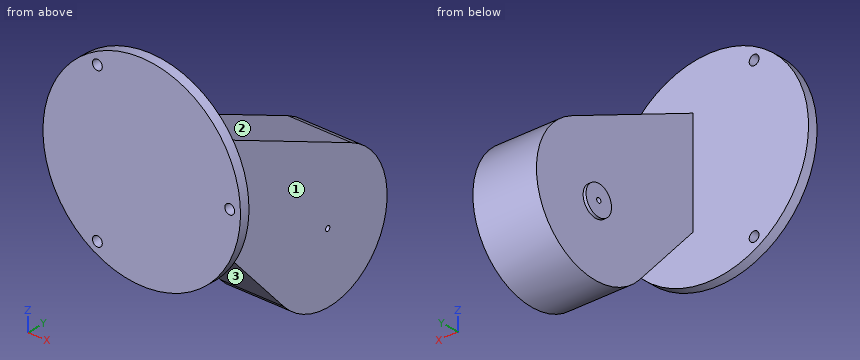
```python
from build123d import *

# Parameters (mm, degrees)
SKETCH_1_R               = 101
EXTRUDE_1_DEPTH          = 10
SKETCH_2_R               = 5
CUT_EXTRUDE_1_DEPTH      = 144.185194765
PATTERN_CIRCULAR_1_COUNT = 3
SKETCH_4_W               = 2.176372913
SKETCH_4_H               = 3.886380203
EXTRUDE_2_DEPTH          = 10
EXTRUDE_3_DEPTH          = 65
CUT_EXTRUDE_2_REACH      = 270.441
SKETCH_6_R               = 2.5
SKETCH_7_R               = 15
EXTRUDE_4_DEPTH          = 3
SKETCH_8_R               = 2.5
CUT_EXTRUDE_3_DEPTH      = 3
SKETCH_9_W               = 6.543349856
SKETCH_9_H               = 10.764234758
CUT_EXTRUDE_4_DEPTH      = 10


with BuildPart() as part:
    # 草图1 → 凸台-拉伸1 (new body)
    with BuildSketch(Plane(origin=(0, 0, 0), x_dir=(1, 0, 0), z_dir=(0, 1, 0))):
        with Locations(Location((0, 0, 0), (0, 0, 270))):
            Circle(SKETCH_1_R)
    extrude(amount=EXTRUDE_1_DEPTH)

    # 草图2 → 切除-拉伸1 (cut, through all)
    with BuildSketch(Plane(origin=(0, 10, 0), x_dir=(1, 0, 0), z_dir=(0, 1, 0))):
        with Locations(Location((90, 0, 0), (0, 0, 270))):
            Circle(SKETCH_2_R)
    cut_extrude_1 = extrude(amount=-CUT_EXTRUDE_1_DEPTH, mode=Mode.SUBTRACT)

    # 阵列(圆周)1: 切除-拉伸1 ×3 about axis
    pattern_circular_1_axis = Axis((-0.221108491, 0, 0), (0, 1, 0))
    for i in range(1, PATTERN_CIRCULAR_1_COUNT):
        add(cut_extrude_1.rotate(pattern_circular_1_axis, i * 360 / PATTERN_CIRCULAR_1_COUNT), mode=Mode.SUBTRACT)

    # 草图4 → 凸台-拉伸2 (add)
    with BuildSketch(Plane(origin=(0, 10, 0), x_dir=(1, 0, 0), z_dir=(0, 1, 0))):
        with Locations((98.327159319, -0.022531505)):
            Rectangle(SKETCH_4_W, SKETCH_4_H)
    extrude(amount=EXTRUDE_2_DEPTH)

    # 草图5 → 凸台-拉伸3 (add)
    with BuildSketch(Plane.ZY.offset(-82.238972862)):
        with BuildLine():
            Line((-119.770908646, 72.705399825), (-51.25005009, 10))
            Line((-51.25005009, 10), (54.128166527, 10))
            Line((54.128166527, 10), (-8.416959639, 152.482035135))
            ThreePointArc((-8.416959639, 152.482035135), (-113.280560411, 181.249471787), (-119.770908646, 72.705399825))
        make_face()
    extrude(amount=EXTRUDE_3_DEPTH)

    # 草图6 → 切除-拉伸2 (cut, up to next)
    with BuildSketch(Plane.ZY.offset(-17.238972862), mode=Mode.PRIVATE) as cut_extrude_2_sk1:
        with Locations((-72.513360124, 124.345733942)):
            Circle(SKETCH_6_R)
    cut_extrude_2_tool1 = extrude(cut_extrude_2_sk1.sketch, amount=-CUT_EXTRUDE_2_REACH, mode=Mode.PRIVATE) & part.part
    add(cut_extrude_2_tool1.solids().sort_by_distance((17.238973, 124.345734, -72.51336))[0], mode=Mode.SUBTRACT)

    # 草图7 → 凸台-拉伸4 (add)
    with BuildSketch(Plane.ZY.offset(-17.238972862)):
        with Locations((-72.513360124, 124.345733942)):
            Circle(SKETCH_7_R)
    extrude(amount=EXTRUDE_4_DEPTH)

    # 草图8 → 切除-拉伸3 (cut)
    with BuildSketch(Plane.ZY.offset(-14.238972862)):
        with Locations((-72.513360124, 124.345733942)):
            Circle(SKETCH_8_R)
    extrude(amount=-CUT_EXTRUDE_3_DEPTH, mode=Mode.SUBTRACT)

    # 草图9 → 切除-拉伸4 (cut)
    with BuildSketch(Plane(origin=(99.415345775, 0, 0), x_dir=(0, 0, -1), z_dir=(1, 0, 0))):
        with Locations((0.262028791, 15.382117379)):
            Rectangle(SKETCH_9_W, SKETCH_9_H)
    extrude(amount=-CUT_EXTRUDE_4_DEPTH, mode=Mode.SUBTRACT)


solid = part.part
```
Read the model definition and answer for the solid it produces. Units are mm, in the model's axes. Face numbers are marked on the shaded views. A direction names the side the tool comes from. Give positions to 0.01 mm unless a question says otherwise; leave off trailing zeros. Loops run counter-clockwise (first coordinate to the right, second up) from the corner with the lowest first, then second, coordinate; pieces in that order, holes last.
Item 1: For the marked faces 1, 2 and 3, determine the directions among +Z, -Z, +X, -X, +Y, -Y from which every point of the face is accessible in a straight line to the end or side of a thin tool.
Item 2: The part is cut by section A-A (x = -45.5). Write down the section's boundary in (y, z), and give its area (3 significant figures).
Item 3: The part is cut by section C-C (x = 69). Write down the section's boundary in (y, z).
Item 4: Each of these flat-tipped pins is pushed along its axis until it touches: pin 1 Ø10 at (y, z) = (37, 50) entering from -X; pin 2 Ø4 at (y, z) = (45, -90) entering from -X; pin 3 Ø2 at (x, y) = (29, 78) entering from +Z. Where does it stop, or does it pass through?
Item 5: The part is cut by section D-D (z = 48). Write down the section's boundary in (x, y).
Item 6: Find the intervals of material crossed by line 1 along X through (y, z) = (111, -38.5); line 2 along Z through (x, y) = (90, 3.5); line 3 along Y through (x, z) = (3, -44), in increasing order.
Item 7: The part is cut by section B-B (z = 0). Write down the section's boundary in (x, y).
Taken from the geometry:
1. face 1: +Z, -Z, +X, +Y
1. face 2: +Z, +X, -X, +Y
1. face 3: -Z, +X, -X
2. outline: (0, -90.17) - (10, -90.17) - (10, -83.13) - (0, -83.13) - close; (0, -73.14) - (10, -73.14) - (10, 73.14) - (0, 73.14) - close; (0, 83.13) - (10, 83.13) - (10, 90.17) - (0, 90.17) - close
2. area: 1,600 mm2
3. outline: (0, -73.76) - (10, -73.76) - (10, -51.25) - (72.71, -119.77) arc R70 ccw (long way) to (152.48, -8.42) - (10, 54.13) - (10, 73.76) - (0, 73.76) - close; hole circle Ø5 at (124.35, -72.51)
4. pin 1: passes through
4. pin 2: stops at x = 17.24
4. pin 3: stops at z = 24.72
5. outline: (-88.87, 0) - (88.87, 0) - (88.87, 10) - (82.24, 10) - (82.24, 23.96) - (17.24, 23.96) - (17.24, 10) - (-88.87, 10) - close
6. line 1: x = 17.24 to 82.24
6. line 2: z = -45.84 to -5, 5 to 45.84
6. line 3: y = 0 to 10
7. outline: (-101, 0) - (85, 0) - (85, 10) - (82.24, 10) - (82.24, 133.31) - (17.24, 133.31) - (17.24, 10) - (-101, 10) - close; (95, 0) - (101, 0) - (101, 10) - (95, 10) - close
